```python
from build123d import *

# Parameters (mm, degrees)
SKETCH1_R           = 4
BOSS_EXTRUDE1_DEPTH = 2
SKETCH2_R           = 5
BOSS_EXTRUDE2_DEPTH = 1.85
FILLET1_R           = 0.15


with BuildPart() as part:
    # Sketch1 → Boss-Extrude1 (new body)
    with BuildSketch(Plane(origin=(0, 0, 0), x_dir=(1, 0, 0), z_dir=(0, 1, 0))):
        with Locations(Location((0, 0, 0), (0, 0, 270))):
            Circle(SKETCH1_R)
        Polygon((2.829016319, 0), (1.41450816, 2.45), (-1.41450816, 2.45), (-2.829016319, 0), (-1.41450816, -2.45), (1.41450816, -2.45), align=None, mode=Mode.SUBTRACT)
    extrude(amount=BOSS_EXTRUDE1_DEPTH)

    # Sketch2 → Boss-Extrude2 (add)
    with BuildSketch(Plane.XZ):
        with Locations(Location((0, 0, 0), (0, 0, 270))):
            Circle(SKETCH2_R)
        Polygon((2.829016319, 0), (1.41450816, 2.45), (-1.41450816, 2.45), (-2.829016319, 0), (-1.41450816, -2.45), (1.41450816, -2.45), align=None, mode=Mode.SUBTRACT)
    extrude(amount=BOSS_EXTRUDE2_DEPTH)

    # Fillet1
    fillet1_edges = [part.edges().sort_by_distance(p)[0] for p in [
        (0, 0, -4),
    ]]
    fillet(fillet1_edges, radius=FILLET1_R)


solid = part.part
```
The listing builds one solid part. Answer for the finished solid, in the listing's coordinates (mm). A direction names the side the tool comes from. Coordinates: 2 decimals unless noted, no trailing zeros. Loops run counter-clockwise (first coordinate to the right, second up) from the corner with the lowest first, then second, coordinate; pieces in that order, holes last. Notation, with made-up numbers: (34.5, 74.25) -> (93.5, 74.25) arc R14 cw to (93.5, 86.25) -> close; hole circle Ø10 at (82.25, 16). An arc over 180 degrees is marked (long way). Return JSON: item names as keys, results as strings. Group by question number.
(1) Which of the six approach directions +Z, -Z, +X, -X, +Y, -Y give full straight-line access (tool end or side, diameter ignored) to faces 1 (the flat face through (-2, -1.85, -2)), 2 (the cylindrical face through (-3.905, 1.062, -0.867)), 3 (the flat face through (-2.112, 0.102, 1.242))?
(2) Determine the mould class of faces 4 (the cylindrical face through (-4.88, -0.91, 1.08)), 5 (the flat face through (-2.13, 0.1, -1.21)), 6 (the flat face through (0, 0, -2.45)), 7 (the flat face through (4, 0, 2)) for opening direction Z: released by +Z, released by -Z, zero draft, split by the parting line, or undercut.
(3) A cutting plane is placed at C-C on y = 1.5. Write down the section's boundary in (x, z).
(4) Find the intervals of material crossed by probe 1 along Z at (x, y) = (-2.25, 1.05); probe 2 along Z at (x, y) = (0.5, -1.2); probe 3 along Y at (x, z) = (-4, 1), in increasing order. Write a range as from..to.
(5) A cutting plane is placed at A-A on y = -0.8. Write down the section's boundary in (x, z), and give its area (3 significant figures).
(6) A cutting plane is placed at B-B on x = 0. Write down the section's boundary in (y, z), and give its area (3 significant figures).
(7) Given pin 1 Ø1 at (x, y) = (4, 1.5) entering from -Z; pin 2 Ø1.5 at (y, z) = (1, 3) entering from +X; pin 3 Ø2 at (x, y) = (-2, -1) entering from -Z; pin 4 Ø0.8 at (x, y) = (0.5, -0.5) entering from -Z, each flat-ended and moving along its own axis, determine where each tip first touches the part or whether it passes through.
The answers:
{
 "1": {"face 1": "+Z, -Z, +X, -X, -Y", "face 2": "+Y", "face 3": "+Y, -Y"},
 "2": {"face 4": "split by the parting line", "face 5": "undercut", "face 6": "undercut", "face 7": "zero draft"},
 "3": {"outline": "circle Ø8 at (0, 0); hole (-2.83, 0) -> (-1.41, -2.45) -> (1.41, -2.45) -> (2.83, 0) -> (1.41, 2.45) -> (-1.41, 2.45) -> close"},
 "4": {"probe 1": "z = -3.31..-1, 1..3.31", "probe 2": "z = -4.97..-2.45, 2.45..4.97", "probe 3": "y = -1.85..0"},
 "5": {"outline": "circle Ø10 at (0, 0); hole (-2.83, 0) -> (-1.41, -2.45) -> (1.41, -2.45) -> (2.83, 0) -> (1.41, 2.45) -> (-1.41, 2.45) -> close", "area": "57.7 mm^2"},
 "6": {"outline": "(-1.85, -5) -> (0, -5) -> (0, -4.15) arc R0.15 cw to (0.15, -4) -> (2, -4) -> (2, -2.45) -> (-1.85, -2.45) -> close; (-1.85, 2.45) -> (2, 2.45) -> (2, 4) -> (0.15, 4) arc R0.15 cw to (0, 4.15) -> (0, 5) -> (-1.85, 5) -> close", "area": "15.6 mm^2"},
 "7": {"pin 1": "stops at z = -1.94", "pin 2": "stops at x = 3.31", "pin 3": "stops at z = -4.9", "pin 4": "stops at z = -5"}
}
